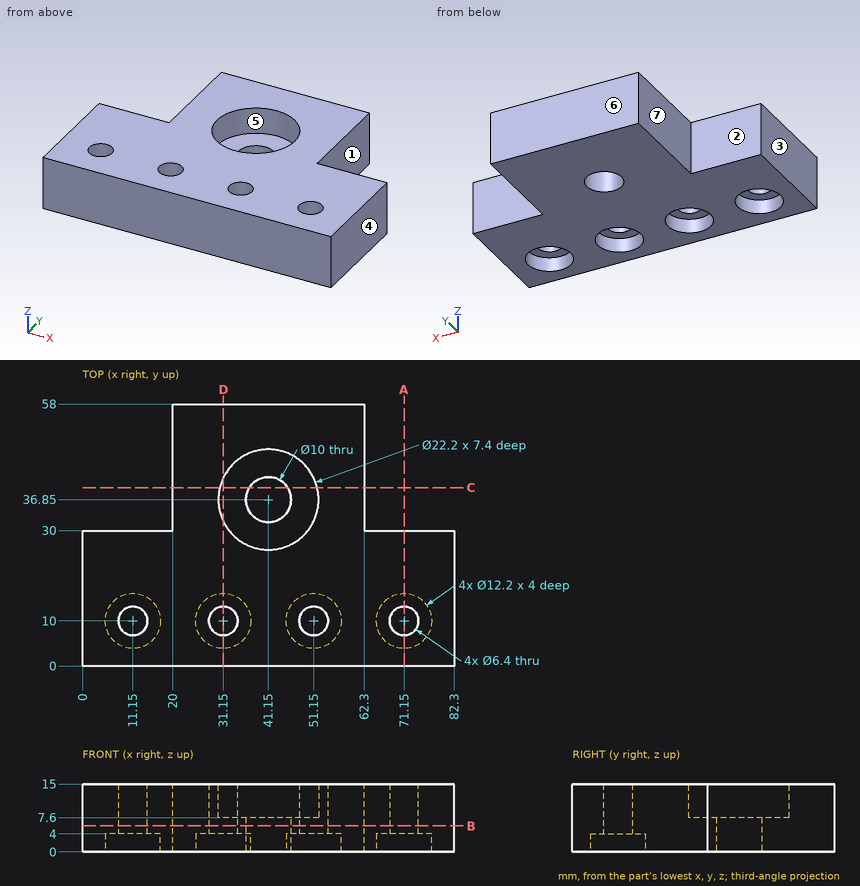
Study the drawing (mm; zero at the part's minimum x, y, z) and answer. A direction names the side the tool comes from. Round coordinates to 2 decimals unless told otherwise and drop trailing zeros. Write each loop counter-clockwise with the first axis right and the second up, starting at its lowest first coordinate (ties: lowest second). Pieces come first, ordered by that corner, then holes. Notation, with made-up numbers: (-9, -6.75) - (35, -6.75) arc R31 ccw to (35, 25.25) - close; hole circle Ø11 at (79, 28.25). An arc over 180 degrees is marked (long way). Use CSV: the item, a comma, the result in double quotes.
Q1. Find section A-A, the plane x = 71.15. Write down the section's boundary in (y, z), then the cut area to 3 significant figures.
Values:
outline,"(0, 0) - (3.9, 0) - (3.9, 4) - (6.8, 4) - (6.8, 15) - (0, 15) - close; (13.2, 4) - (16.1, 4) - (16.1, 0) - (30, 0) - (30, 15) - (13.2, 15) - close"
area,"331 mm²"
Q2. Find section D-D, the plane x = 31.15. Write down the section's boundary in (y, z), then the cut area to 4 significant figures.
Values:
outline,"(0, 0) - (3.9, 0) - (3.9, 4) - (6.8, 4) - (6.8, 15) - (0, 15) - close; (13.2, 4) - (16.1, 4) - (16.1, 0) - (58, 0) - (58, 15) - (41.67, 15) - (41.67, 7.6) - (32.03, 7.6) - (32.03, 15) - (13.2, 15) - close"
area,"679.5 mm²"
Q3. Find section B-B, the plane z = 5.75. Write down the section's boundary in (x, y).
Values:
outline,"(0, 0) - (82.3, 0) - (82.3, 30) - (62.3, 30) - (62.3, 58) - (20, 58) - (20, 30) - (0, 30) - close; hole circle Ø6.4 at (11.15, 10); hole circle Ø6.4 at (31.15, 10); hole circle Ø10 at (41.15, 36.85); hole circle Ø6.4 at (51.15, 10); hole circle Ø6.4 at (71.15, 10)"
Q4. Find section C-C, the plane y = 39.5. Write down the section's boundary in (x, z), then the cut area to 3 significant figures.
Values:
outline,"(20, 0) - (36.91, 0) - (36.91, 7.6) - (30.37, 7.6) - (30.37, 15) - (20, 15) - close; (45.39, 0) - (62.3, 0) - (62.3, 15) - (51.93, 15) - (51.93, 7.6) - (45.39, 7.6) - close"
area,"411 mm²"
Q5. A tool of negligible diameter and unlimited length cuts with its end or side. For the marked faces 1, 2 and 3, from which of +Z, -Z, +X, -X, +Y, -Y can it reach the whole face along a straight path? Write none if from no direction.
Values:
face 1,"+Z, -Z, +X, +Y"
face 2,"+Z, -Z, -X, +Y"
face 3,"+Z, -Z, -X, +Y, -Y"
Q6. Determine the mould class of the marked faces 4, 5, 6 and 7 for opening direction X: +X half, -X half, draft (parallel to the pull), parting line (faces both ways), or undercut.
Values:
face 4,"+X half"
face 5,"undercut"
face 6,"draft"
face 7,"-X half"
Q7. Each of these flat-tipped pins is pushed along its axis until it touches: pin 1 Ø4.5 at (y, z) = (44, 4.5) entering from +X; pin 2 Ø3 at (x, z) = (70, 7) entering from +Y; pin 3 Ø13 at (x, y) = (41.15, 36.85) entering from +Z. Where does it stop, or does it pass through?
Values:
pin 1,"stops at x = 62.3"
pin 2,"stops at y = 30"
pin 3,"stops at z = 7.6"
Q8. Straight lines are drawn through the part: line 1 along X through (y, z) = (10, 1.75); line 2 along X through (y, z) = (10, 9); line 3 along Y through (x, z) = (71.5, 1.75). For each, find the intervals that lie inside material, in ascending order.
Values:
line 1,"x = 0 to 5.05, 17.25 to 25.05, 37.25 to 45.05, 57.25 to 65.05, 77.25 to 82.3"
line 2,"x = 0 to 7.95, 14.35 to 27.95, 34.35 to 47.95, 54.35 to 67.95, 74.35 to 82.3"
line 3,"y = 0 to 3.91, 16.09 to 30"
